from build123d import *

# Parameters (mm, degrees)
F0_W     = 350
F0_H     = 200
F0_R     = 7.5
F1_DEPTH = 10


with BuildPart() as f1:
    # F0 (on Front) → F1 (new body)
    with BuildSketch(Plane.XZ):
        Rectangle(F0_W, F0_H)
        with Locations((-58.5, 10)):
            Circle(F0_R, mode=Mode.SUBTRACT)
        with Locations((17.5, 10)):
            Circle(F0_R, mode=Mode.SUBTRACT)
        with Locations((70, 10)):
            Circle(F0_R, mode=Mode.SUBTRACT)
    extrude(amount=F1_DEPTH)


solid = f1.part
CAD build for the part. Positions are in the model's coordinates, mm. Coordinates: 2 decimals unless noted, no trailing zeros. Loops run counter-clockwise (first coordinate to the right, second up) from the corner with the lowest first, then second, coordinate; pieces in that order, holes last. Notation, with made-up numbers: (59.5, 60.5) - (74.5, 60.5) arc R31 cw to (74.5, 99.5) - close; hole circle Ø7 at (29.5, 57). An arc over 180 degrees is marked (long way). Write item = value, one per line. Start each with the question number.
Q1. Cut at C-C, the plane x = -58. List the corners of the cut face in (y, z), then the cut area to 3 significant figures.
Q2. Pull direction X, two halves, no side cores. Call faces 1 (the flat face through (-2, 0, 1)), 2 (the cylindrical face through (11.548, -4.93, 5.436)), 3 (the cylindrical face through (-64.452, -4.93, 5.436)), 4 (the flat face through (175, -5, -1)): pulls with the +X half, pulls with the -X half, needs draft (parallel to the pull), parting line crosses it, or undercut.
Q3. Flat gauge pin, fed straight in: pin 1 Ø9 at (x, z) = (-58.5, 10) entering from -Y. Where does the tip first touch, or does it go through?
Q4. Cut at A-A, the plane z = 10. List the corners of the cut face in (x, y).
Q5. Cut at B-B, the plane x = 70. List the corners of the cut face in (y, z), then the cut area to 3 significant figures.
Q6. Drill centre lines: L1, parallel to Z at x = 17.5, y = -3.5; L2, parallel to X at y = -1, z = 16. Where is each one in solid material? Low to high.
Computed:
q1.outline = (-10, -100) - (0, -100) - (0, 2.52) - (-10, 2.52) - close; (-10, 17.48) - (0, 17.48) - (0, 100) - (-10, 100) - close
q1.area = 1,850 mm²
q2.face_1 = needs draft
q2.face_2 = undercut
q2.face_3 = undercut
q2.face_4 = pulls with the +X half
q3.pin_1 = through
q4.outline = (-175, -10) - (-66, -10) - (-66, 0) - (-175, 0) - close; (-51, -10) - (10, -10) - (10, 0) - (-51, 0) - close; (25, -10) - (62.5, -10) - (62.5, 0) - (25, 0) - close; (77.5, -10) - (175, -10) - (175, 0) - (77.5, 0) - close
q5.outline = (-10, -100) - (0, -100) - (0, 2.5) - (-10, 2.5) - close; (-10, 17.5) - (0, 17.5) - (0, 100) - (-10, 100) - close
q5.area = 1,850 mm²
q6.L1 = -100 to 2.5, 17.5 to 100
q6.L2 = -175 to -63, -54 to 13, 22 to 65.5, 74.5 to 175
